Autodesk Inventor part; units mm, degrees
ref_plane "YZ Plane" through (0, 0, 0) normal (1, 0, 0) x (0, 1, 0)
ref_plane "XZ Plane" through (0, 0, 0) normal (0, 1, 0) x (-1, 0, 0)
ref_plane "XY Plane" through (0, 0, 0) normal (0, 0, 1) x (1, 0, 0)
sketch "Эскиз1" plane through (0, 0, 0) normal (0, 1, 0) x (-1, 0, 0)
  circle A0 centre (0, 0) radius 50
  dimension "d0" = 100
extrude "Выдавливание1" add sketch "Эскиз1" along normal blind 130
sketch "Эскиз2" plane through (0, 130, 0) normal (0, 1, 0) x (1, 0, 0)
  circle A0 centre (0, 0) radius 5
  dimension "d3" = 10
extrude "Выдавливание2" add sketch "Эскиз2" along normal blind 30
fillet "Сопряжение1" radius 5 2 edges at (50, 130, 0) (50, 0, 0)
properties part number "МоторКолес"
Could you check a few things on this model? Use its own coordinates, in mm. A direction names the side the tool comes from. Give positions to 0.01 mm unless a question says otherwise; leave off trailing zeros. Loops run counter-clockwise (first coordinate to the right, second up) from the corner with the lowest first, then second, coordinate; pieces in that order, holes last. Notation, with made-up numbers: (23.5, 75) -> (33.5, 75) arc R21 cw to (33.5, 87) -> close; hole circle Ø3 at (69, -19). An arc over 180 degrees is marked (long way). Return JSON: item names as keys, results as strings.
Item 1: If we section it at D-D on y = 134.5: List the corners of the cut face in (x, z) for me.
Geometry results:
{"outline": "circle Ø10 at (0, 0)"}
Item 2: If we section it at B-B on z = 0: List the corners of the cut face in (x, y) for me.
Geometry results:
{"outline": "(-50, 5) arc R5 ccw to (-45, 0) -> (45, 0) arc R5 ccw to (50, 5) -> (50, 125) arc R5 ccw to (45, 130) -> (5, 130) -> (5, 160) -> (-5, 160) -> (-5, 130) -> (-45, 130) arc R5 ccw to (-50, 125) -> close"}
Item 3: I need wall thicknesses on L1, parallel to Y at x = 17, z = -24; L2, parallel to X at y = 103, z = 1; L3, parallel to Z at x = 30, y = 103. Which ranges of each line are inside material? Lowest first, please. Write a range as from..to.
Geometry results:
{"L1": "y = 0..130", "L2": "x = -49.99..49.99", "L3": "z = -40..40"}
Item 4: If we section it at A-A on x = 0: List the corners of the cut face in (y, z) for me.
Geometry results:
{"outline": "(0, -45) arc R5 ccw to (5, -50) -> (125, -50) arc R5 ccw to (130, -45) -> (130, -5) -> (160, -5) -> (160, 5) -> (130, 5) -> (130, 45) arc R5 ccw to (125, 50) -> (5, 50) arc R5 ccw to (0, 45) -> close"}
Item 5: I'm going to push flat-ended pins straight in: pin 1 (10 mm diameter, centred on x = -15, y = 118.5, fed in from +Z); pin 2 (2 mm diameter, centred on y = 63.5, z = 39.5, fed in from -X); pin 3 (6 mm diameter, centred on y = 82.5, z = -39, fed in from +X). Where does each tip first touch, or does it pass through?
Geometry results:
{"pin 1": "stops at z = 48.99", "pin 2": "stops at x = -31.9", "pin 3": "stops at x = 34.7"}
Item 6: Which directions (+Z, -Z, +X, -X, +Y, -Y) give clear straight access to the entire face, cutting with the end or side of a thin tool? Please do faces 1 (the cylindrical face through (-1.08, 144.79, -4.88)), 2 (the flat face through (0, 160, 0)).
Geometry results:
{"face 1": "+Y", "face 2": "+Z, -Z, +X, -X, +Y"}
Item 7: If we section it at C-C on y = 58.5: List the corners of the cut face in (x, z) for me.
Geometry results:
{"outline": "circle Ø100 at (0, 0)"}
